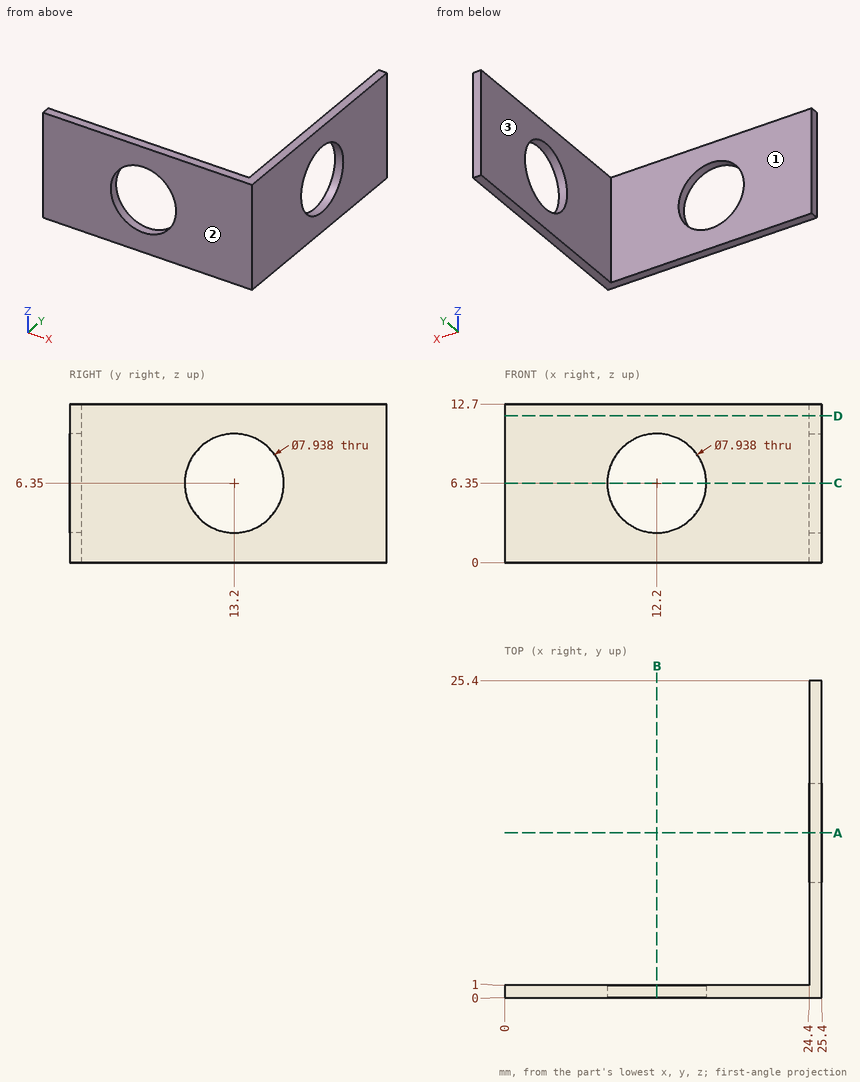
Here's the drawing with two shaded views (mm, measured from the low corner). I have some questions. Coordinates: 2 decimals unless noted, no trailing zeros. Loops run counter-clockwise (first coordinate to the right, second up) from the corner with the lowest first, then second, coordinate; pieces in that order, holes last. Notation, with made-up numbers: M -0.75,-6.75 L 37.25,-6.75 A27 ccw 37.25,19.25 Z; hole C 24.25,84 d1. An arc over 180 degrees is marked long. Return JSON: item names as keys, results as strings. Group by question number.
Item 1: Imagine slicing it at A-A (y = 13.2). Please give me the cut outline in (x, z).
Item 2: Imagine slicing it at C-C (z = 6.35). Please give me the cut outline in (x, y).
Item 3: Imagine slicing it at B-B (x = 12.2). Please give me the cut outline in (y, z).
Item 4: Imagine slicing it at D-D (z = 11.75). Please give me the cut outline in (x, y).
Item 5: If I drill on L1, parallel to Y at x = 25.15, z = 6.35; L2, parallel to Z at x = 12.2, y = 0.5; L3, parallel to Y at x = 6.25, z = 4, over which ranges is the centre line in solid material (lowest first)? Write a range as from..to.
Item 6: Thinking about a two-plate mould opening in Y: for the marked faces 1, 2 and 3, which applies, released by +Y, released by -Y, zero draft, split by the parting line, or undercut?
Item 7: I'm going to push flat-ended pins straight in: pin 1 Ø4 at (x, z) = (19.5, 11) entering from +Y; pin 2 Ø3 at (x, z) = (9, 9.5) entering from -Y. Where does each tip first touch, or does it pass through?
Verdict:
{
 "1": {"outline": "M 24.4,0 L 25.4,0 L 25.4,2.38 L 24.4,2.38 Z; M 24.4,10.32 L 25.4,10.32 L 25.4,12.7 L 24.4,12.7 Z"},
 "2": {"outline": "M 0,0 L 8.23,0 L 8.23,1 L 0,1 Z; M 16.17,0 L 25.4,0 L 25.4,9.23 L 24.4,9.23 L 24.4,1 L 16.17,1 Z; M 24.4,17.17 L 25.4,17.17 L 25.4,25.4 L 24.4,25.4 Z"},
 "3": {"outline": "M 0,0 L 1,0 L 1,2.38 L 0,2.38 Z; M 0,10.32 L 1,10.32 L 1,12.7 L 0,12.7 Z"},
 "4": {"outline": "M 0,0 L 25.4,0 L 25.4,25.4 L 24.4,25.4 L 24.4,1 L 0,1 Z"},
 "5": {"L1": "y = 0..9.23, 17.17..25.4", "L2": "z = 0..2.38, 10.32..12.7", "L3": "y = 0..1"},
 "6": {"face 1": "released by +Y", "face 2": "released by -Y", "face 3": "zero draft"},
 "7": {"pin 1": "stops at y = 1", "pin 2": "stops at y = 0"}
}
